Geometry: see drawing. Coordinates: mm, zero at the bounding-box minimum. Round coordinates to 2 decimals unless told otherwise and drop trailing zeros. Loops run counter-clockwise (first coordinate to the right, second up) from the corner with the lowest first, then second, coordinate; pieces in that order, holes last. Notation, with made-up numbers: (-27, 35.5) - (12, 35.5) arc R23 ccw to (12, 59.5) - close; hole circle Ø5 at (89.5, 61.5). An arc over 180 degrees is marked (long way). Write item = value, one per line. Start each with the question number.
Item 1: First-contact query: pin 1 (1.5 mm diameter, centred on x = 23, z = 1.5, fed in from +Y); pin 2 (0.9 mm diameter, centred on y = 1.5, z = 2, fed in from +X); pin 3 (0.9 mm diameter, centred on y = 2, z = 1, fed in from -X). Flat tips, straight axial feed; report the tip coordinate or a pass-through.
Item 2: Line query: line 1 (Y direction, x = 23.25, z = 1.2); line 2 (X direction, y = 20, z = 1.15); line 3 (Y direction, x = 8.5, z = 0.4). Output: solid intervals per line, ascending. Write a range as from..to.
Item 3: Section B-B (x = 10.5). Return loops of the section in (y, z).
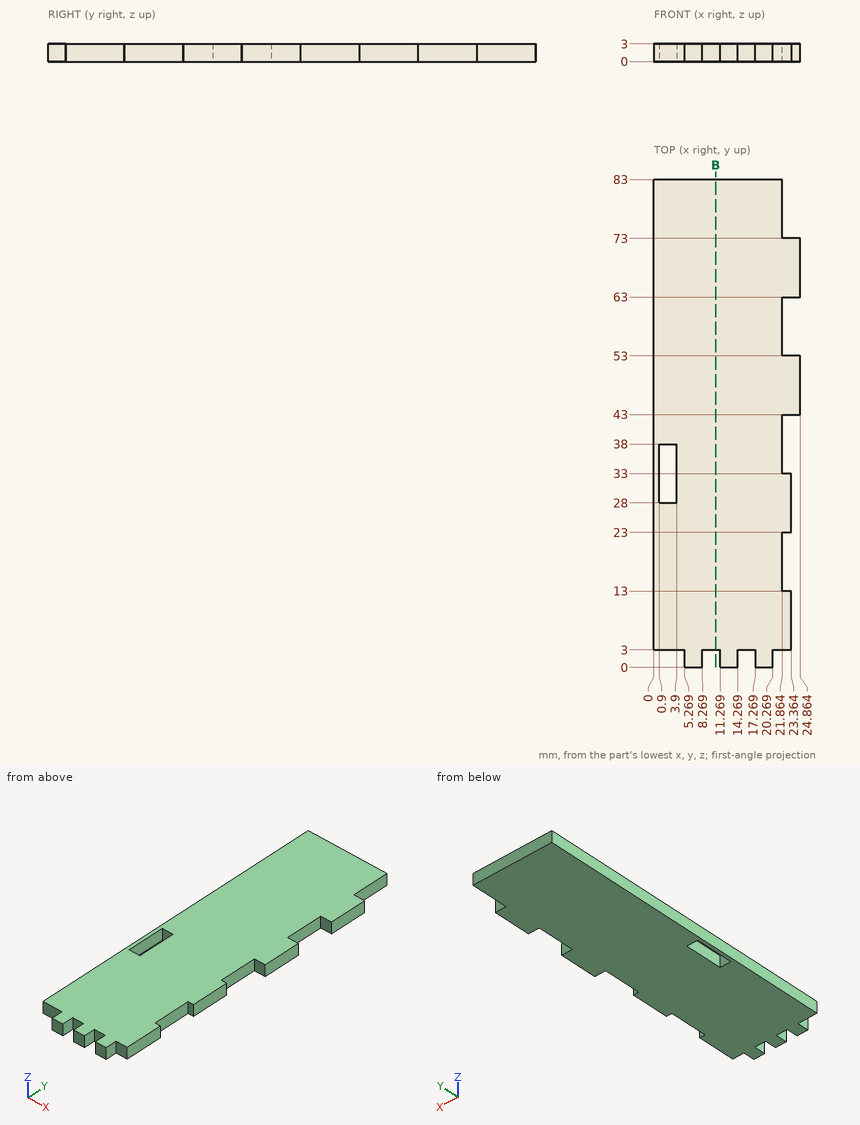
Taken from the geometry:
q1.pin_1 = 73
q1.pin_2 = 20.27
q1.pin_3 = 5.27
q2.line_1 = 3..13, 23..33, 43..53, 63..73
q2.line_2 = 0..21.86
q2.line_3 = 3..83
q3.outline = (3, 0) - (83, 0) - (83, 3) - (3, 3) - close
